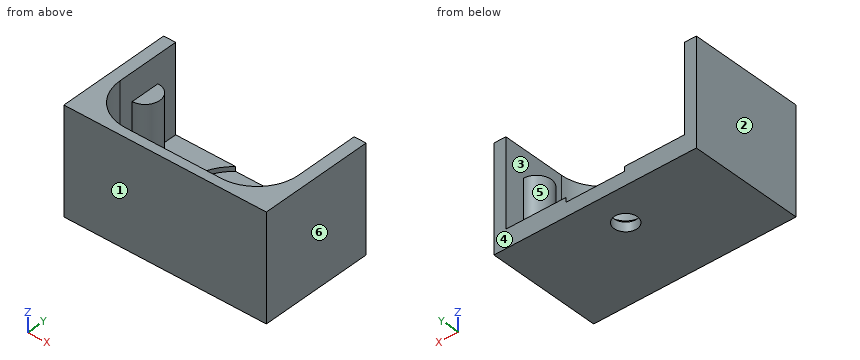
Autodesk Inventor part; units mm, degrees
ref_plane "YZ Plane" through (0, 0, 0) normal (1, 0, 0) x (0, 1, 0)
ref_plane "XZ Plane" through (0, 0, 0) normal (0, 1, 0) x (-1, 0, 0)
ref_plane "XY Plane" through (0, 0, 0) normal (0, 0, 1) x (1, 0, 0)
sketch "Sketch1" plane through (0, 0, 0) normal (0, 0, 1) x (1, 0, 0)
  line L0 (9.7, 0) -> (-9.7, 0)
  line L1 (-9.7, 0) -> (-9.7, 11.4)
  line L2 (-9.7, 11.4) -> (9.7, 11.4)
  line L3 (9.7, 11.4) -> (9.7, 0)
  line L4 (-9.7, 6) -> (-9.7, 0)
  line L5 (-9.7, 0) -> (9.7, 0)
  line L6 (9.7, 0) -> (9.7, 6)
  arc A0 (-9.7, 6) -> (-9.7, 9.2) centre (-9.7, 7.6) ccw
  arc A1 (9.7, 9.2) -> (9.7, 6) centre (9.7, 7.6) ccw
  line L7 (6.5, 0) -> (-6.5, 0)
  line L8 (-6.5, 0) -> (-6.5, 3)
  line L9 (-6.5, 3) -> (6.5, 3)
  line L10 (6.5, 3) -> (6.5, 0)
  line L11 (2.9833, 3.65) -> (-2.9833, 3.65)
  line L12 (-3.1721, 11.4) -> (3.1721, 11.4)
  arc A2 (-3.1721, 11.4) -> (-2.9833, 3.65) centre (0, 7.6) ccw
  arc A3 (2.9833, 3.65) -> (3.1721, 11.4) centre (0, 7.6) ccw
  circle A4 centre (0, 7.6) radius 1.25
  line L13 (11, -1) -> (-11, -1)
  line L14 (-11, -1) -> (-11, 11.4)
  line L15 (-11, 11.4) -> (11, 11.4)
  line L16 (11, 11.4) -> (11, -1)
  point P0 (0, 0)
  dimension "d0" = 19.4
  dimension "d1" = 11.4
  dimension "d3" = 13
  dimension "d5" = 2.5
  dimension "d6" = 22
  dimension "d7" = 12.4
extrude "Extrusion1" add sketch "Sketch1" along normal blind 10 contours L3 L15 L16 L13 L14 L1 L0
extrude "Extrusion3" add sketch "Sketch1" along normal blind 8.5 contours A1 L3 | L1 A0
extrude "Extrusion4" add sketch "Sketch1" along normal blind 1.5 contours L0 L10 L9 L8 L1 A0 L2 A2 L11 A3 L3 A1 | L0 L8 L9 L10 | A3 L11 A2 L2
chamfer "Chamfer1" distance 0.5 angle 45 1 edges at (-1.25, 7.6, 1.5)
fillet "Fillet1" radius 4.5 2 edges at (-9.7, 0, 5.75) (9.7, 0, 5.75)
extrude "Extrusion6" add sketch "Sketch1" along normal blind 2 contours L0 L10 L9 L8 L1 A0 L2 A2 L11 A3 L3 A1 | L0 L8 L9 L10
move faces "Move1" translate (0, 0, 1.5) faces at (-1.7333, -0.6667, 10)
sketch "Sketch2" plane through (-11, -1, 0) normal (0, -1, 0) x (1, 0, 0)
  line L0 (22, 0) -> (22, 11.5)
  line L1 (0, 0) -> (22, 0)
  line L2 (22, 0) -> (22, 1)
  line L3 (22, 1) -> (0, 1)
  line L4 (0, 1) -> (0, 0)
  line L5 (5, 0) -> (4.6249, 0)
  line L6 (4.6249, 1) -> (5, 1)
  line L7 (0, 0) -> (22, 0)
  line L8 (17, 0) -> (17, 1)
  line L9 (5, 0) -> (5, 1)
  line L10 (1, 0) -> (1, 1)
  line L11 (21, 0) -> (21, 1)
  point P0 (11, 0)
  point P1 (0, 0.5)
  point P2 (4.9955, 0.5057)
  point P3 (5, 0.5)
  point P4 (21, 0.5)
  point P5 (1, 0)
  dimension "d28" = 1
  dimension "d30" = 5
  dimension "d31" = 5
  dimension "d32" = 1
  dimension "d33" = 1
extrude "Extrusion7" add sketch "Sketch2" along normal blind 1.5 contours L1 L11 L3 L0 | L1 L9 L3 L8 | L1 L4 L3 L10
move faces "Move2" translate (0, 1.5, 0) faces at (-10.6667, -2.5, 0.6667) (2, -2.5, 0.3333) (10.6667, -2.5, 0.6667)
properties part number "MotorHolder"
The listing builds one solid part. Answer for the finished solid, in the listing's coordinates (mm). Face numbers are marked on the shaded views. A direction names the side the tool comes from. Round coordinates to 2 decimals unless told otherwise and drop trailing zeros. Order: outer loops, then holes, each group sorted by start corner. A loop starts at its lowest first (then second) coordinate and runs counter-clockwise, first axis right, second up. Notation, with made-up numbers: (50.5, 38.5) - (65.5, 38.5) arc R18 cw to (65.5, 71.5) - close; hole circle Ø10 at (8.5, -3). An arc over 180 degrees is marked (long way). Put each result on its own line as item: value. Start each with the question number.
(1) Given P1, Ø5, axis at x = 2.5, z = 7, coming from the +Y side; P2, Ø2, axis at x = -4.5, y = 7.5, coming from the +Z side; P3, Ø4, axis at x = 0, y = 7.6, coming from the +Z side, each flat-ended and moving along its own axis, determine where each tip first touches the part or whether it passes through.
(2) For the marked faces 5 and 6, determine the directions among +Z, -Z, +X, -X, +Y, -Y from which every point of the face is accessible in a straight line to the end or side of a thin tool.
(3) Straight lines are drawn through the part: probe 1 along X at (y, z) = (5, 10.75); probe 2 along Y at (x, z) = (0, 0.4); probe 3 along Z at (x, y) = (2.75, 3). For each, find the intervals that lie inside material, in ascending order. Write a range as from..to.
(4) Determine the mould class of the marked faces 1, 2, 3 and 4 for opening direction Y: released by +Y, released by -Y, zero draft, split by the parting line, or undercut.
(5) Find section D-D (y = 10.75). Give the vertices of the cut face in (x, z).
(6) Find section A-A (y = 7.6). Give the vertices of the cut face in (x, z).
(7) Find section C-C (z = 2.25). Give the vertices of the cut face in (x, y), plus the area to 3 significant figures.
(8) Find section B-B (x = 0). Give the vertices of the cut face in (y, z), plus the area to 3 significant figures.
Reply:
1. P1: y = 0
1. P2: z = 2
1. P3: z = 1.5
2. face 5: +Z
2. face 6: +Z, -Z, +X, +Y, -Y
3. probe 1: -11..-9.7, 9.7..11
3. probe 2: -1..6.35, 8.85..11.4
3. probe 3: 0..2
4. face 1: released by -Y
4. face 2: zero draft
4. face 3: undercut
4. face 4: released by +Y
5. outline: (-11, 0) - (11, 0) - (11, 11.5) - (9.7, 11.5) - (9.7, 2) - (3.82, 2) - (3.82, 1.5) - (-3.82, 1.5) - (-3.82, 2) - (-9.7, 2) - (-9.7, 11.5) - (-11, 11.5) - close
6. outline: (-11, 0) - (-1.25, 0) - (-1.25, 1) - (-1.75, 1.5) - (-4.95, 1.5) - (-4.95, 2) - (-8.1, 2) - (-8.1, 8.5) - (-9.7, 8.5) - (-9.7, 11.5) - (-11, 11.5) - close; (1.25, 0) - (11, 0) - (11, 11.5) - (9.7, 11.5) - (9.7, 8.5) - (8.1, 8.5) - (8.1, 2) - (4.95, 2) - (4.95, 1.5) - (1.75, 1.5) - (1.25, 1) - close
7. outline: (-11, -1) - (11, -1) - (11, 11.4) - (9.7, 11.4) - (9.7, 9.2) arc R1.6 ccw to (9.7, 6) - (9.7, 4.5) arc R4.5 cw to (5.2, 0) - (-5.2, 0) arc R4.5 cw to (-9.7, 4.5) - (-9.7, 6) arc R1.6 ccw to (-9.7, 9.2) - (-9.7, 11.4) - (-11, 11.4) - close
7. area: 68.4 mm^2
8. outline: (-1, 0) - (6.35, 0) - (6.35, 1) - (5.85, 1.5) - (3.65, 1.5) - (3.65, 2) - (0, 2) - (0, 11.5) - (-1, 11.5) - close; (8.85, 0) - (11.4, 0) - (11.4, 1.5) - (9.35, 1.5) - (8.85, 1) - close
8. area: 26.4 mm^2
